Verification items for the finished model (mm, model axes). Face numbers are marked on the shaded views. A direction names the side the tool comes from. Coordinates: 2 decimals unless noted, no trailing zeros. Loops run counter-clockwise (first coordinate to the right, second up) from the corner with the lowest first, then second, coordinate; pieces in that order, holes last. Notation, with made-up numbers: (-33, 53) - (-25, 53) arc R23 ccw to (-25, 88) - close; hole circle Ø9 at (-26.75, 38). An arc over 180 degrees is marked (long way). Answer as CSV lines item,"result". Start each with the question number.
1. Cross-section at A-A (x = 7.25). Enter the section's corners in (y, z) (3 decimals), plus the area to 4 significant figures.
2. Gauge pin test, flat ends, axial feed: P1, Ø3.5, axis at x = 6.5, y = -8, coming from the +Z side; P2, Ø3.5, axis at x = 2.5, y = -2, coming from the +Z side; P3, Ø10, axis at x = 5.5, y = -2, coming from the -Z side; P4, Ø0.5, axis at x = 15.5, z = 0.5, coming from the -Y side (3 decimals). Record the tip position at first contact, or that the pin passes through.
3. Set-up check for the marked faces 4, 5, 6 and 7: record each of +Z, -Z, +X, -X, +Y, -Y from which the full face is reachable in a straight line by a thin tool's end or side.
4. Cross-section at C-C (y = 0). Enter the section's corners in (x, z), plus the area to 3 significant figures.
5. Cross-section at D-D (z = 1.25). Enter the section's corners in (x, y) (3 decimals).
6. Material ranges on line 1 (Y direction, x = 16, z = 3.25) (3 decimals); line 2 (Y direction, x = 8.25, z = 1.45) (3 decimals); line 3 (X direction, y = -3.25, z = 3), recorded low to high. Write a range as [from, to].
7. Release check for a two-part mould opening along Y. For the marked faces 1, 2 and 3 record: pulls with the +Y half, pulls with the -Y half, needs draft (parallel to the pull), parting line crosses it, or undercut.
8. Cross-section at B-B (z = 3.8). Enter the section's corners in (x, y) (3 decimals), plus the area to 3 significant figures.
```python
from build123d import *

# Parameters (mm, degrees)
F1_DEPTH  = 9.075
F3_DEPTH  = 1.3
F6_DEPTH  = 6.05
F7_W      = 15
F7_H      = 2
F8_DEPTH  = 4.601
F9_W      = 1
F9_H      = 0.6
F10_DEPTH = 3


with BuildPart() as f1:
    # F0 (on Front) → F1 (new body, symmetric)
    with BuildSketch(Plane.XZ):
        with BuildLine():
            Line((-3.0842823463, 3), (-6.0842823463, 0))
            Line((-6.0842823463, 0), (15.0370379973, 0))
            Line((15.0370379973, 0), (17.0763778255, 2.0393398282))
            ThreePointArc((17.0763778255, 2.0393398282), (17.0763778255, 4.1606601718), (14.9550574819, 4.1606601718))
            Line((14.9550574819, 4.1606601718), (13.7943973101, 3))
            Line((13.7943973101, 3), (-3.0842823463, 3))
        make_face()
    extrude(amount=F1_DEPTH, both=True)

    # F2 (on face) → F3 (join)
    with BuildSketch(Plane.XZ.offset(9.075)):
        with BuildLine():
            ThreePointArc((17.0763778255, 2.0393398282), (17.4015369525, 2.5259748515), (17.5157176537, 3.1))
            ThreePointArc((17.5157176537, 3.1), (16.5897428022, 4.4858192988), (14.9550574819, 4.1606601718))
            ThreePointArc((14.9550574819, 4.1606601718), (14.9550574819, 2.0393398282), (17.0763778255, 2.0393398282))
        make_face()
    extrude(amount=F3_DEPTH)

    # F4: F1 across plane


with BuildPart() as f1_1:
    add(f1.part)
    add(f1.part.mirror(Plane.XZ))

    # F5 (on Front) → F6 (cut, symmetric)
    with BuildSketch(Plane.XZ):
        Polygon((12.7943973101, 2), (13.7943973101, 3), (-3.0842823463, 3), (-4.0842823463, 2), align=None)
    extrude(amount=F6_DEPTH, both=True, mode=Mode.SUBTRACT)

    # F7 (on Top) → F8 (cut, through all)
    with BuildSketch(Plane.XY):
        with Locations((11.4157176537, -5.05)):
            Rectangle(F7_W, F7_H)
        with Locations((11.4157176537, 5.05)):
            Rectangle(F7_W, F7_H)
    extrude(amount=F8_DEPTH, mode=Mode.SUBTRACT)

    # F9 (on Top) → F10 (join)
    with BuildSketch(Plane.XY):
        with Locations((15.4550574819, 9.375)):
            Rectangle(F9_W, F9_H)
        with Locations((15.4550574819, -9.375)):
            Rectangle(F9_W, F9_H)
    extrude(amount=F10_DEPTH)


solid = f1_1.part
```
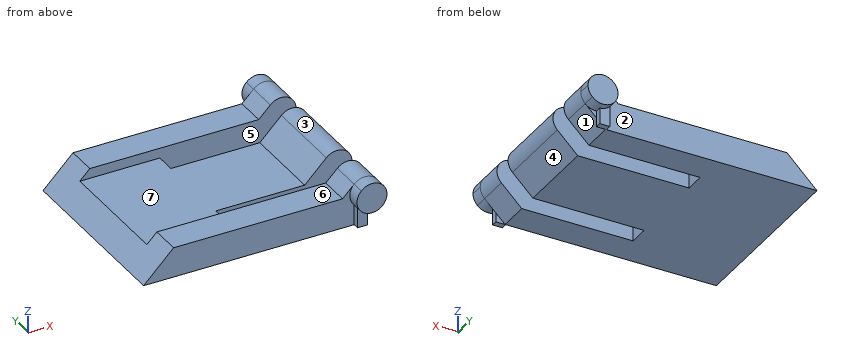
Values follow:
1,outline,"(-9.075, 0) - (-6.05, 0) - (-6.05, 3) - (-9.075, 3) - close; (-4.05, 0) - (4.05, 0) - (4.05, 2) - (-4.05, 2) - close; (6.05, 0) - (9.075, 0) - (9.075, 3) - (6.05, 3) - close"
1,area,"34.35 mm²"
2,P1,"stops at z = 3"
2,P2,"stops at z = 2"
2,P3,"stops at z = 0"
2,P4,"stops at y = -9.675"
3,face 4,"-Z, +X"
3,face 5,"+Z, +X"
3,face 6,"+Z, -X, +Y, -Y"
3,face 7,"+Z, -X"
4,outline,"(-6.08, 0) - (15.04, 0) - (17.08, 2.04) arc R1.5 ccw to (14.96, 4.16) - (12.79, 2) - (-4.08, 2) - close"
4,area,"50.4 mm²"
5,outline,"(-4.834, -9.075) - (14.955, -9.075) - (14.955, -9.675) - (15.955, -9.675) - (15.955, -9.075) - (16.287, -9.075) - (16.287, -6.05) - (3.916, -6.05) - (3.916, -4.05) - (16.287, -4.05) - (16.287, 4.05) - (3.916, 4.05) - (3.916, 6.05) - (16.287, 6.05) - (16.287, 9.075) - (15.955, 9.075) - (15.955, 9.675) - (14.955, 9.675) - (14.955, 9.075) - (-4.834, 9.075) - close"
6,line 1,"y = [-10.375, -6.05], [-4.05, 4.05], [6.05, 10.375]"
6,line 2,"y = [-9.075, -6.05], [-4.05, 4.05], [6.05, 9.075]"
6,line 3,"x = [13.79, 17.51]"
7,face 1,"undercut"
7,face 2,"pulls with the +Y half"
7,face 3,"needs draft"
8,outline,"(14.594, -9.075) - (14.689, -9.075) - (14.689, -10.375) - (17.342, -10.375) - (17.342, -6.05) - (14.594, -6.05) - close; (14.594, -4.05) - (17.342, -4.05) - (17.342, 4.05) - (14.594, 4.05) - close; (14.594, 6.05) - (17.342, 6.05) - (17.342, 10.375) - (14.689, 10.375) - (14.689, 9.075) - (14.594, 9.075) - close"
8,area,"45.8 mm²"
